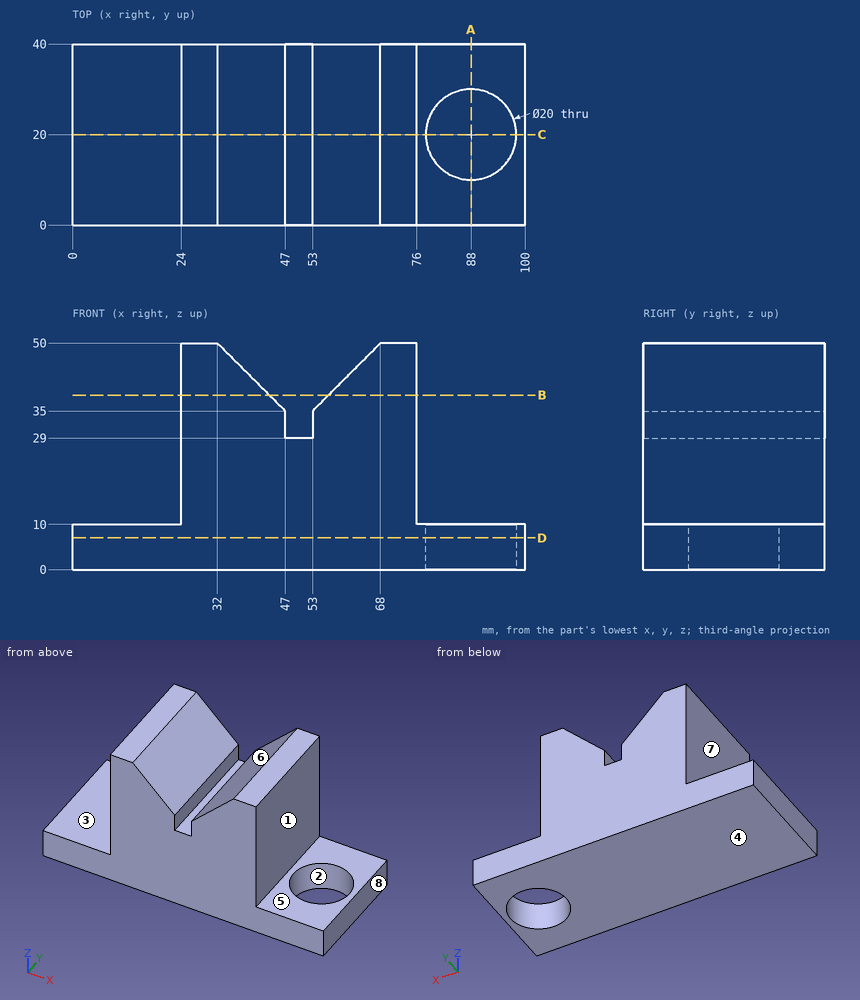
Could you check a few things on this drawing? It's one solid part, dimensions in mm from its lowest x, y, z. A direction names the side the tool comes from. Round coordinates to 2 decimals unless told otherwise and drop trailing zeros. Loops run counter-clockwise (first coordinate to the right, second up) from the corner with the lowest first, then second, coordinate; pieces in that order, holes last. Notation, with made-up numbers: (8.5, -25) -> (33.5, -25) arc R27 ccw to (33.5, -4) -> close; hole circle Ø8 at (-3.5, 63.5). An arc over 180 degrees is marked (long way). Answer as CSV lines item,"result".
1. Thinking about a two-plate mould opening in X: for the marked faces 1, 2 and 3, which applies, released by +X, released by -X, zero draft, split by the parting line, or undercut?
Final values:
face 1,"released by +X"
face 2,"undercut"
face 3,"zero draft"
2. If we section it at D-D on z = 7: Please give me the cut outline in (x, y), plus the area to 3 significant figures.
Final values:
outline,"(0, 0) -> (100, 0) -> (100, 40) -> (0, 40) -> close; hole circle Ø20 at (88, 20)"
area,"3,690 mm^2"
3. If we section it at C-C on y = 20: Please give me the cut outline in (x, z), plus the area to 3 significant figures.
Final values:
outline,"(0, 0) -> (78, 0) -> (78, 10) -> (76, 10) -> (76, 50) -> (68, 50) -> (53, 35) -> (53, 29) -> (47, 29) -> (47, 35) -> (32, 50) -> (24, 50) -> (24, 10) -> (0, 10) -> close; (98, 0) -> (100, 0) -> (100, 10) -> (98, 10) -> close"
area,"2,530 mm^2"
4. For pin 1 (12 mm diameter, centred on y = 17.5, z = 41.5, fed in from +X); pin 2 (1.5 mm diameter, centred on x = 16.5, y = 34.5, fed in from +Z); pin 3 (12 mm diameter, centred on y = 13, z = 25, fed in from -X), each with a flat end and sliding along its axis, tell me the tip position at first contact or that it passes through.
Final values:
pin 1,"stops at x = 76"
pin 2,"stops at z = 10"
pin 3,"stops at x = 24"
5. If we section it at B-B on z = 38.5: Please give me the cut outline in (x, y), plus the area to 3 significant figures.
Final values:
outline,"(24, 0) -> (43.5, 0) -> (43.5, 40) -> (24, 40) -> close; (56.5, 0) -> (76, 0) -> (76, 40) -> (56.5, 40) -> close"
area,"1,560 mm^2"
6. Which directions (+Z, -Z, +X, -X, +Y, -Y) give clear straight access to the entire face, cutting with the end or side of a thin tool? Please do the marked faces 4, 5, 6, 7 and 8.
Final values:
face 4,"-Z, +X, -X, +Y, -Y"
face 5,"+Z, +X, +Y, -Y"
face 6,"+Z, +Y, -Y"
face 7,"+Z, -X, +Y, -Y"
face 8,"+Z, -Z, +X, +Y, -Y"
7. If we section it at A-A on x = 88: Please give me the cut outline in (y, z), plus the area to 3 significant figures.
Final values:
outline,"(0, 0) -> (10, 0) -> (10, 10) -> (0, 10) -> close; (30, 0) -> (40, 0) -> (40, 10) -> (30, 10) -> close"
area,"200 mm^2"
8. If I drill on L1, parallel to Y at x = 88, z = 7.25; L2, parallel to X at y = 4.5, z = 35; L3, parallel to Z at x = 14, y = 30.5, over which ranges is the centre line in solid material (lowest first)?
Final values:
L1,"y = 0 to 10, 30 to 40"
L2,"x = 24 to 47, 53 to 76"
L3,"z = 0 to 10"
